from build123d import *

# Parameters (mm, degrees)
SKETCH1_R               = 3.175
BOSS_EXTRUDE1_DEPTH     = 190.5
CUT_EXTRUDE1_DEPTH      = 191.552909319
CUT_EXTRUDE1_DEPTH_BACK = 191.552909319
SKETCH2_R               = 1.63195
CUT_EXTRUDE2_START      = 2.54
SKETCH2_3_W             = 6.35
SKETCH2_3_H             = 15.5259893
SKETCH2_3_R             = 1.63195
SKETCH2_3_H_2           = 21.77390706
CUT_EXTRUDE2_DEPTH      = 189.012909422


with BuildPart() as part:
    # Sketch1 → Boss-Extrude1 (new body)
    with BuildSketch(Plane(origin=(0, 0, 0), x_dir=(0, 0, -1), z_dir=(1, 0, 0))):
        Circle(SKETCH1_R)
    extrude(amount=BOSS_EXTRUDE1_DEPTH)

    # Sketch2 → Cut-Extrude1 (cut, two sides: drawn at the far end of the back side and taken through both)
    with BuildSketch(Plane(origin=(0, 0, 0), x_dir=(1, 0, 0), z_dir=(0, 1, 0)).offset(-CUT_EXTRUDE1_DEPTH_BACK)):
        with Locations(Location((52.38623, 0, 0), (0, 0, 270))):
            Circle(SKETCH2_R)
        with Locations(Location((68.26377, 0, 0), (0, 0, 270))):
            Circle(SKETCH2_R)
        with Locations(Location((129.4, 0, 0), (0, 0, 270))):
            Circle(SKETCH2_R)
        with Locations(Location((111.9, 0, 0), (0, 0, 270))):
            Circle(SKETCH2_R)
        with Locations(Location((171.45, 0, 0), (0, 0, 270))):
            Circle(SKETCH2_R)
    extrude(amount=CUT_EXTRUDE1_DEPTH + CUT_EXTRUDE1_DEPTH_BACK, mode=Mode.SUBTRACT)

    # Sketch2_3 → Cut-Extrude2 (cut, through all)
    # profile 1 of 5: a face of its own
    with BuildSketch(Plane(origin=(0, 0, 0), x_dir=(1, 0, 0), z_dir=(0, 1, 0)).offset(CUT_EXTRUDE2_START)):
        with Locations((52.38623, 0)):
            Rectangle(SKETCH2_3_W, SKETCH2_3_H)
        with Locations(Location((52.38623, 0, 0), (0, 0, 270))):
            Circle(SKETCH2_3_R, mode=Mode.SUBTRACT)
    # profile 2 of 5: a face of its own
    with BuildSketch(Plane(origin=(0, 0, 0), x_dir=(1, 0, 0), z_dir=(0, 1, 0)).offset(CUT_EXTRUDE2_START)):
        with Locations((68.26377, 0)):
            Rectangle(SKETCH2_3_W, SKETCH2_3_H)
        with Locations(Location((68.26377, 0, 0), (0, 0, 270))):
            Circle(SKETCH2_3_R, mode=Mode.SUBTRACT)
    # profile 3 of 5: a face of its own
    with BuildSketch(Plane(origin=(0, 0, 0), x_dir=(1, 0, 0), z_dir=(0, 1, 0)).offset(CUT_EXTRUDE2_START)):
        with Locations((129.4, 0)):
            Rectangle(SKETCH2_3_W, SKETCH2_3_H)
        with Locations(Location((129.4, 0, 0), (0, 0, 270))):
            Circle(SKETCH2_3_R, mode=Mode.SUBTRACT)
    # profile 4 of 5: a face of its own
    with BuildSketch(Plane(origin=(0, 0, 0), x_dir=(1, 0, 0), z_dir=(0, 1, 0)).offset(CUT_EXTRUDE2_START)):
        with Locations((171.45, 0)):
            Rectangle(SKETCH2_3_W, SKETCH2_3_H_2)
        with Locations(Location((171.45, 0, 0), (0, 0, 270))):
            Circle(SKETCH2_3_R, mode=Mode.SUBTRACT)
    # profile 5 of 5: a face of its own
    with BuildSketch(Plane(origin=(0, 0, 0), x_dir=(1, 0, 0), z_dir=(0, 1, 0)).offset(CUT_EXTRUDE2_START)):
        with Locations((111.9, 0)):
            Rectangle(SKETCH2_3_W, SKETCH2_3_H)
    extrude(amount=CUT_EXTRUDE2_DEPTH, mode=Mode.SUBTRACT)


solid = part.part
Design review of the part built by this model. Coordinates are the model's own, in mm. A direction names the side the tool comes from. Round coordinates to 2 decimals unless told otherwise and drop trailing zeros. Loops run counter-clockwise (first coordinate to the right, second up) from the corner with the lowest first, then second, coordinate; pieces in that order, holes last. Notation, with made-up numbers: M 46.25,8.25 L 73.25,8.25 A19 ccw 73.25,32.25 Z; hole C -30,-38 d3. An arc over 180 degrees is marked long. Answer as a JSON object with one key per item and string values.
Item 1: Wall thickness on L1, parallel to X at y = -0.8, z = 0; L2, parallel to X at y = -2, z = 0.5; L3, parallel to Z at x = 129.4, y = 0.1: over which ranges is each line inside the solid? List them lowest first. Write a range as from..to.
Answer sheet:
{"L1": "x = 0..50.75, 54.02..66.63, 69.9..110.27, 113.53..127.77, 131.03..169.82, 173.08..190.5", "L2": "x = 0..50.83, 53.94..66.71, 69.82..110.35, 113.45..127.85, 130.95..169.9, 173..190.5", "L3": "z = -3.17..-1.63, 1.63..3.17"}
Item 2: We need section A-A on x = 129.4. Give the boundary of the cut face in (y, z) (3 decimals), and give its area (3 significant figures).
Answer sheet:
{"outline": "M -2.723,-1.632 A3.175 ccw 2.54,-1.905 L 2.54,-1.632 Z; M -2.723,1.632 L 2.54,1.632 L 2.54,1.905 A3.175 ccw Z", "area": "11.8 mm^2"}
Item 3: Machinability: for faces 5 (the flat face through (67.5, 2.54, 1.7)), 6 (the cylindrical face through (69.882, -0.359, -0.212)), which of the approach directions +Z, -Z, +X, -X, +Y, -Y give a long, thin tool a straight path to every point of the face, cutting with its end or side? Answer none if there is none.
Answer sheet:
{"face 5": "+Z, -Z, +Y", "face 6": "+Y, -Y"}
Item 4: We need section B-B on y = 0. Give the boundary of the cut face in (x, z) (3 decimals).
Answer sheet:
{"outline": "M 0,-3.175 L 190.5,-3.175 L 190.5,3.175 L 0,3.175 Z; hole C 52.386,0 d3.264; hole C 68.264,0 d3.264; hole C 111.9,0 d3.264; hole C 129.4,0 d3.264; hole C 171.45,0 d3.264"}
Item 5: Clearance check with flat-ended pins moving along their axes: P1, Ø1, axis at y = 1, z = 1, coming from the -X side; P2, Ø1.1, axis at x = 51, z = -1, coming from the +Y side; P3, Ø1.5, axis at x = 106, z = 1, coming from the +Y side. State where each tip first meets the part, or that it passes through.
Answer sheet:
{"P1": "stops at x = 0", "P2": "stops at y = 2.54", "P3": "stops at y = 3.17"}
Item 6: The part is to be moulded in two halves that separate along Z. For faces 1 (the cylindrical face through (173.07, -0.36, -0.21)), 2 (the cylindrical face through (54.004, -0.359, -0.212)), 3 (the cylindrical face through (93.92, -3.1, 0.69)), 4 (the flat face through (0, 0, 0)), say which applies: pulls with the +Z half, pulls with the -Z half, needs draft (parallel to the pull), parting line crosses it, or undercut.
Answer sheet:
{"face 1": "undercut", "face 2": "undercut", "face 3": "parting line crosses it", "face 4": "needs draft"}
Item 7: We need section D-D on x = 106.5. Give the boundary of the cut face in (y, z) (3 decimals), and give its area (3 significant figures).
Answer sheet:
{"outline": "C 0,0 d6.35", "area": "31.7 mm^2"}
Item 8: We need section C-C on z = 0. State how many separate pieces and enclosed holes the cut face has, and give its area (3 significant figures).
Answer sheet:
{"separate pieces": "6", "enclosed holes": "0", "area": "1,100 mm^2"}
